Geometry check sheet. Reference: the model listing, model coordinates, mm. A direction names the side the tool comes from. Coordinates: 2 decimals unless noted, no trailing zeros. Loops run counter-clockwise (first coordinate to the right, second up) from the corner with the lowest first, then second, coordinate; pieces in that order, holes last.
Autodesk Inventor part; units mm, degrees
ref_plane "YZ Plane" through (0, 0, 0) normal (1, 0, 0) x (0, 1, 0)
ref_plane "XZ Plane" through (0, 0, 0) normal (0, 1, 0) x (-1, 0, 0)
ref_plane "XY Plane" through (0, 0, 0) normal (0, 0, 1) x (1, 0, 0)
sketch "스케치1" plane through (0, 0, 0) normal (0, 0, 1) x (1, 0, 0)
  line L0 (-6.05, -3) -> (-6.05, 3)
  line L1 (6.05, -3) -> (-6.05, -3)
  line L2 (6.05, 3) -> (6.05, -3)
  line L3 (-6.05, 3) -> (6.05, 3)
  line L4 (6.05, 3) -> (6.05, -3)
  line L5 (6.05, -3) -> (43, -3)
  line L6 (43, 3) -> (43, -3)
  line L7 (6.05, 3) -> (43, 3)
  circle A0 centre (20, 0) radius 1.35
  circle A1 centre (-20, 0) radius 1.35
  line L8 (-6.05, -3) -> (-6.05, 3)
  line L9 (-6.05, 3) -> (-43, 3)
  line L10 (-43, -3) -> (-43, 3)
  line L11 (-6.05, -3) -> (-43, -3)
  line L12 (-43, -32.95) -> (-37, -32.95)
  line L13 (-37, -32.95) -> (-37, -3)
  line L14 (-37, -3) -> (-43, -3)
  line L15 (-43, -3) -> (-43, -32.95)
  line L16 (-43, -45.05) -> (-43, -32.95)
  line L17 (-37, -45.05) -> (-43, -45.05)
  line L18 (-37, -32.95) -> (-37, -45.05)
  line L19 (-43, -32.95) -> (-37, -32.95)
  line L20 (-37, -45.05) -> (-43, -45.05)
  line L21 (-43, -45.05) -> (-43, -75)
  line L22 (-43, -75) -> (-37, -75)
  line L23 (-37, -75) -> (-37, -45.05)
  line L24 (37, -32.95) -> (43, -32.95)
  line L25 (43, -32.95) -> (43, -3)
  line L26 (43, -3) -> (37, -3)
  line L27 (37, -3) -> (37, -32.95)
  line L28 (37, -45.05) -> (37, -32.95)
  line L29 (43, -45.05) -> (37, -45.05)
  line L30 (43, -32.95) -> (43, -45.05)
  line L31 (37, -32.95) -> (43, -32.95)
  line L32 (43, -45.05) -> (37, -45.05)
  line L33 (37, -45.05) -> (37, -75)
  line L34 (37, -75) -> (43, -75)
  line L35 (43, -75) -> (43, -45.05)
  line L36 (-37, -3) -> (37, -3)
  line L37 (37, -3) -> (37, -75)
  line L38 (37, -75) -> (-37, -75)
  line L39 (-37, -75) -> (-37, -3)
  line L40 (6, -3) -> (-6, -3)
  line L41 (-6, -3) -> (-6, 3)
  line L42 (-6, 3) -> (6, 3)
  line L43 (6, 3) -> (6, -3)
  line L44 (37, -33) -> (43, -33)
  line L45 (43, -33) -> (43, -45)
  line L46 (43, -45) -> (37, -45)
  line L47 (37, -45) -> (37, -33)
  line L48 (-37, -33) -> (-43, -33)
  line L49 (-43, -33) -> (-43, -45)
  line L50 (-43, -45) -> (-37, -45)
  line L51 (-37, -45) -> (-37, -33)
  point P0 (0, 0)
  dimension "d0" = 12
  dimension "d1" = 6
  dimension "d2" = 6
  dimension "d3" = 12
  dimension "d4" = 6
  dimension "d5" = 12
extrude "돌출1" add sketch "스케치1" along normal blind 6 contours L1 L5 L27 L28 L33 L38 L23 L18 L13 L11 | L41 L3 L43 L1 | L18 L50 L16 L48 | L44 L30 L46 L28
sketch "스케치2" plane through (-6, 3, 0) normal (0, 1, 0) x (1, 0, 0)
  circle A0 centre (34, -3.1) radius 1.35
  circle A1 centre (-22, -3.1) radius 1.35
  circle A2 centre (34, -3.1) radius 1.35
  circle A3 centre (-22, -3.1) radius 1.35
  point P0 (6, 0)
extrude "돌출2" cut sketch "스케치2" against normal blind 20
sketch "스케치3" plane through (-43, -45, 0) normal (-1, 0, 0) x (0, 0, 1)
  circle A0 centre (3.1, -5.05) radius 1.35
  circle A1 centre (3.1, -5.05) radius 1.35
  point P0 (0, 45)
extrude "돌출3" cut sketch "스케치3" against normal blind 20
sketch "스케치4" plane through (43, -45, 0) normal (1, 0, 0) x (0, 0, -1)
  circle A0 centre (-3, -5.05) radius 1.35
  circle A1 centre (-3, -5.05) radius 1.35
  point P0 (0, 45)
extrude "돌출4" cut sketch "스케치4" against normal blind 20
sketch "스케치5" plane through (0, 0, 6) normal (0, 0, 1) x (1, 0, 0)
  line L0 (37, -48.7) -> (23, -48.7)
  line L1 (37, -51.4) -> (23, -51.4)
  line L2 (-37, -51.4) -> (-23, -51.4)
  line L3 (-37, -48.7) -> (-23, -48.7)
  line L4 (-26.65, -3) -> (-26.65, -17)
  line L5 (-29.35, -3) -> (-29.35, -17)
  line L6 (29.35, -3) -> (29.35, -17)
  line L7 (26.65, -3) -> (26.65, -17)
  line L8 (31, -51.4) -> (31, -48.7)
  line L9 (-31, -51.4) -> (-31, -48.7)
  line L10 (29.35, -9) -> (26.65, -9)
  line L11 (-26.65, -9) -> (-29.35, -9)
  line L12 (25.4, -7.9) -> (30.6, -7.9)
  line L13 (30.6, -7.9) -> (30.6, -10.1)
  line L14 (30.6, -10.1) -> (25.4, -10.1)
  line L15 (25.4, -10.1) -> (25.4, -7.9)
  line L16 (25.4, -7.9) -> (30.6, -10.1) construction
  line L17 (30.6, -7.9) -> (25.4, -10.1) construction
  line L18 (29.9, -47.45) -> (32.1, -47.45)
  line L19 (32.1, -47.45) -> (32.1, -52.65)
  line L20 (32.1, -52.65) -> (29.9, -52.65)
  line L21 (29.9, -52.65) -> (29.9, -47.45)
  line L22 (29.9, -47.45) -> (32.1, -52.65) construction
  line L23 (32.1, -47.45) -> (29.9, -52.65) construction
  line L24 (-30.6, -7.9) -> (-25.4, -7.9)
  line L25 (-25.4, -7.9) -> (-25.4, -10.1)
  line L26 (-25.4, -10.1) -> (-30.6, -10.1)
  line L27 (-30.6, -10.1) -> (-30.6, -7.9)
  line L28 (-30.6, -7.9) -> (-25.4, -10.1) construction
  line L29 (-25.4, -7.9) -> (-30.6, -10.1) construction
  line L30 (-32.1, -47.45) -> (-29.9, -47.45)
  line L31 (-29.9, -47.45) -> (-29.9, -52.65)
  line L32 (-29.9, -52.65) -> (-32.1, -52.65)
  line L33 (-32.1, -52.65) -> (-32.1, -47.45)
  line L34 (-32.1, -47.45) -> (-29.9, -52.65) construction
  line L35 (-29.9, -47.45) -> (-32.1, -52.65) construction
  point P0 (0, 0)
  point P1 (28, -9)
  point P2 (31, -50.05)
  point P3 (-28, -9)
  point P4 (-31, -50.05)
  dimension "d14" = 5.2
  dimension "d15" = 2.2
  dimension "d16" = 2.2
  dimension "d17" = 5.2
  dimension "d18" = 5.2
  dimension "d19" = 2.2
  dimension "d20" = 2.2
  dimension "d21" = 5.2
extrude "돌출5" cut sketch "스케치5" against normal blind 20
sketch "스케치6" plane through (0, 0, 6) normal (0, 0, 1) x (1, 0, 0)
  line L0 (-32.1, -52.65) -> (-32.1, -47.45)
  line L1 (-32.1, -47.45) -> (-29.9, -47.45)
  line L2 (-29.9, -47.45) -> (-29.9, -52.65)
  line L3 (-29.9, -52.65) -> (-32.1, -52.65)
  line L4 (29.9, -52.65) -> (29.9, -47.45)
  line L5 (29.9, -47.45) -> (32.1, -47.45)
  line L6 (32.1, -47.45) -> (32.1, -52.65)
  line L7 (32.1, -52.65) -> (29.9, -52.65)
  line L8 (-30.6, -7.9) -> (-25.4, -7.9)
  line L9 (-25.4, -7.9) -> (-25.4, -10.1)
  line L10 (-25.4, -10.1) -> (-30.6, -10.1)
  line L11 (-30.6, -10.1) -> (-30.6, -7.9)
  line L12 (30.6, -10.1) -> (25.4, -10.1)
  line L13 (25.4, -10.1) -> (25.4, -7.9)
  line L14 (25.4, -7.9) -> (30.6, -7.9)
  line L15 (30.6, -7.9) -> (30.6, -10.1)
  line L16 (37, -75) -> (37, -45)
  line L17 (37, -45) -> (43, -45)
  line L18 (43, -45) -> (43, -33)
  line L19 (43, -33) -> (37, -33)
  line L20 (37, -33) -> (37, -3)
  line L21 (37, -3) -> (6, -3)
  line L22 (6, -3) -> (6, 3)
  line L23 (6, 3) -> (-6, 3)
  line L24 (-6, 3) -> (-6, -3)
  line L25 (-6, -3) -> (-37, -3)
  line L26 (-37, -3) -> (-37, -33)
  line L27 (-37, -33) -> (-43, -33)
  line L28 (-43, -33) -> (-43, -45)
  line L29 (-43, -45) -> (-37, -45)
  line L30 (-37, -45) -> (-37, -75)
  line L31 (-37, -75) -> (37, -75)
  circle A0 centre (6, -3) radius 1
  circle A1 centre (-6, -3) radius 1
  circle A2 centre (37, -33) radius 1
  circle A3 centre (37, -45) radius 1
  circle A4 centre (-37, -33) radius 1
  circle A5 centre (-37, -45) radius 1
  point P0 (0, 0)
  point P1 (38, -45)
  point P2 (37, -46)
  point P3 (-37, -46)
  point P4 (-38, -45)
  point P5 (6, -2)
  point P6 (7, -3)
  dimension "d24" = 2
  dimension "d25" = 2
  dimension "d26" = 2
  dimension "d27" = 2
  dimension "d28" = 2
  dimension "d29" = 2
extrude "돌출6" cut sketch "스케치6" against normal through all contours A3 L17 L16 | L30 L29 A5 | A2 L20 L19 | L19 L20 A2 | A4 L26 L27 | L27 L26 A4 | A0 L22 L21 | A1 L24 L25 | L25 L24 A1 picked at (36.339, -44.9727) picked at (-37.1584, -44.3574) picked at (5.6614, -3.5683)
properties part number "overhead" material "PMMA 플라스틱"
1) Access from +Z, -Z, +X, -X, +Y, -Y to the whole of each face (thin tool, end or side, straight path). Record for faces 1 (the flat face through (-41, -45, 3)), 2 (the flat face through (37, -61, 3)), 3 (the flat face through (-29.9, -49, 2)).
Data:
face 1: +Z, -Z, -X, -Y
face 2: +Z, -Z, +X, -Y
face 3: +Z, -Z
2) Section check B-B on y = -14. Record the cut outline in (x, z), and give its area (3 significant figures).
Data:
outline: (-37, 0) - (37, 0) - (37, 6) - (-37, 6) - close; hole circle Ø2.7 at (-28, 3.1); hole circle Ø2.7 at (28, 3.1)
area: 433 mm2
3) Section check A-A on x = 28. Record the cut outline in (y, z).
Data:
outline: (-75, 0) - (-10.1, 0) - (-10.1, 1.75) - (-17, 1.75) - (-17, 4.45) - (-10.1, 4.45) - (-10.1, 6) - (-75, 6) - close; (-7.9, 0) - (-3, 0) - (-3, 1.75) - (-7.9, 1.75) - close; (-7.9, 4.45) - (-3, 4.45) - (-3, 6) - (-7.9, 6) - close; hole circle Ø2.7 at (-50.05, 3)
4) Material ranges on probe 1 along X at (y, z) = (-15, 3.1); probe 2 along Z at (x, y) = (27, -50); probe 3 along X at (y, z) = (-5, 2.45), recorded low to high.
Data:
probe 1: x = -37 to -29.35, -26.65 to 26.65, 29.35 to 37
probe 2: z = 0 to 1.65, 4.35 to 6
probe 3: x = -37 to -29.18, -26.82 to 26.82, 29.18 to 37
5) Mould release check, pull along Y, two halves, no side actions. Record for faces 4 (the flat face through (28, -17, 3)), 5 (the flat face through (-31, -52.65, 3)), 6 (the cylindrical face through (-36.27, -44.317, 3.042)), 7 (the cylindrical face through (29.288, -13.502, 2.694)): +Y half, -Y half, draft (parallel to the pull), parting line (faces both ways), or undercut.
Data:
face 4: +Y half
face 5: undercut
face 6: undercut
face 7: draft
6) Depth check by flat-ended pin: pin 1 (2.5 mm diameter, centred on y = -50.05, z = 3, fed in from +X); pin 2 (10 mm diameter, centred on x = -2, y = -43, fed in from -Z); pin 3 (2.5 mm diameter, centred on y = -9, z = 2.5, fed in from -X); pin 4 (3 mm diameter, centred on y = -50.05, z = 3, fed in from +X). Enter the tip coordinate at first touch or a pass-through.
Data:
pin 1: stops at x = 23
pin 2: stops at z = 0
pin 3: stops at x = -37
pin 4: stops at x = 37
